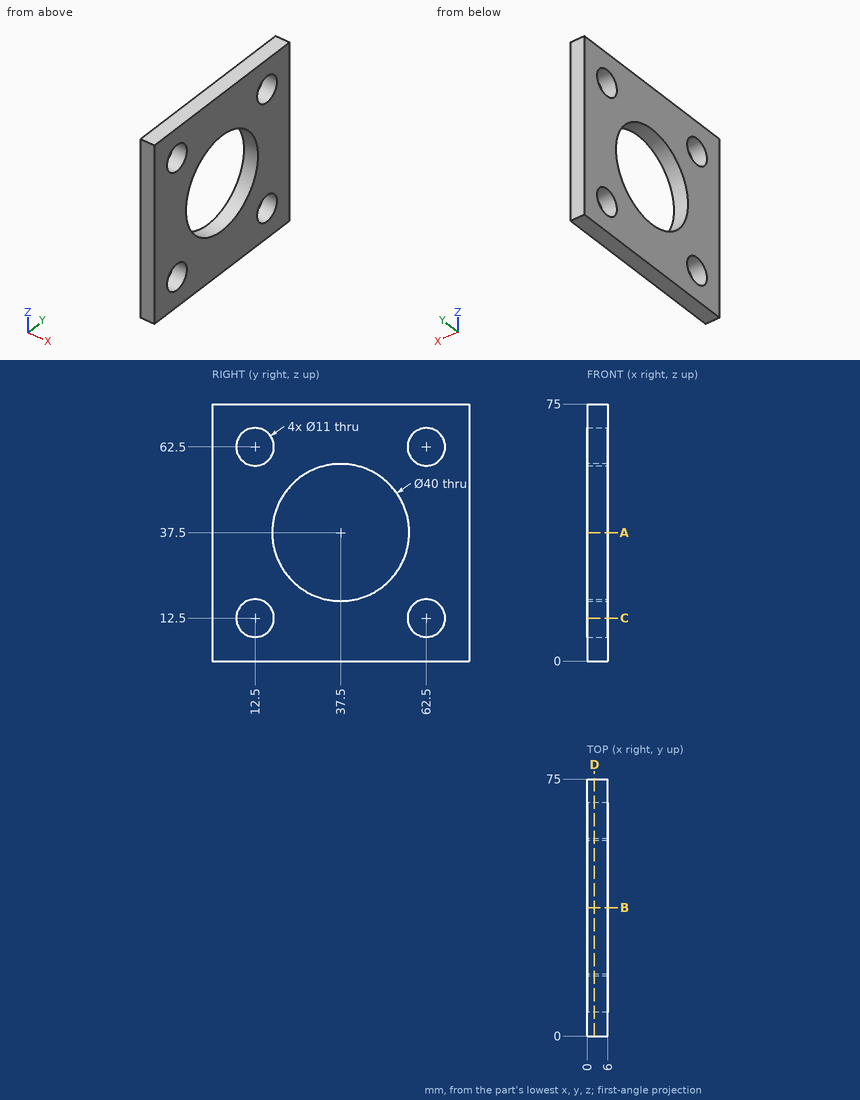
Part print with two shaded views. Sizes in mm from the minimum x, y, z corner. Coordinates: 2 decimals unless noted, no trailing zeros. Loops run counter-clockwise (first coordinate to the right, second up) from the corner with the lowest first, then second, coordinate; pieces in that order, holes last. Notation, with made-up numbers: (39.5, 64) -> (96.5, 64) arc R30 ccw to (96.5, 101) -> close; hole circle Ø5 at (78, -4). An arc over 180 degrees is marked (long way). Answer as a JSON object with one key per item and string values.
Q1. Probe probe 1 along Y at (x, z) = (3.9, 12.5); probe 2 along Y at (x, z) = (2.3, 37.5); probe 3 along Z at (x, y) = (3.8, 64). List the from-to ranges inside material, lowest first.
Report:
{"probe 1": "y = 0 to 7, 18 to 57, 68 to 75", "probe 2": "y = 0 to 17.5, 57.5 to 75", "probe 3": "z = 0 to 7.21, 17.79 to 57.21, 67.79 to 75"}
Q2. Flat gauge pin, fed straight in: P1, Ø6.5, axis at y = 62.5, z = 12.5, coming from the +X side. Where does the tip first touch, or does it go through?
Report:
{"P1": "passes through"}
Q3. Cut at D-D (x = 2.1). List the corners of the cut face in (y, z), and give its area (3 significant figures).
Report:
{"outline": "(0, 0) -> (75, 0) -> (75, 75) -> (0, 75) -> close; hole circle Ø11 at (12.5, 12.5); hole circle Ø11 at (12.5, 62.5); hole circle Ø40 at (37.5, 37.5); hole circle Ø11 at (62.5, 12.5); hole circle Ø11 at (62.5, 62.5)", "area": "3,990 mm2"}
Q4. Cut at C-C (z = 12.5). List the corners of the cut face in (x, y), and give its area (3 significant figures).
Report:
{"outline": "(0, 0) -> (6, 0) -> (6, 7) -> (0, 7) -> close; (0, 18) -> (6, 18) -> (6, 57) -> (0, 57) -> close; (0, 68) -> (6, 68) -> (6, 75) -> (0, 75) -> close", "area": "318 mm2"}
Q5. Cut at A-A (z = 37.5). List the corners of the cut face in (x, y).
Report:
{"outline": "(0, 0) -> (6, 0) -> (6, 17.5) -> (0, 17.5) -> close; (0, 57.5) -> (6, 57.5) -> (6, 75) -> (0, 75) -> close"}
